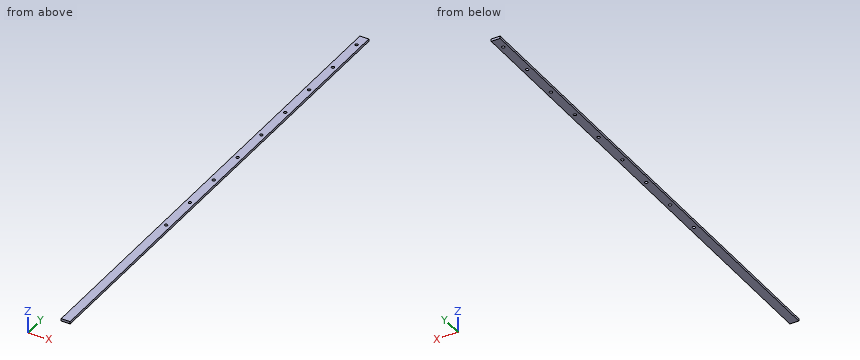
from build123d import *

# Parameters (mm, degrees)
SKETCH1_W           = 18
SKETCH1_H           = 1003
BOSS_EXTRUDE1_DEPTH = 5
SKETCH2_R           = 3
CUT_EXTRUDE1_DEPTH  = 5
LPATTERN1_COUNT     = 9
LPATTERN1_PITCH     = 80


with BuildPart() as part:
    # Sketch1 → Boss-Extrude1 (new body)
    with BuildSketch(Plane.XY):
        Rectangle(SKETCH1_W, SKETCH1_H)
    extrude(amount=BOSS_EXTRUDE1_DEPTH)

    # Sketch2 → Cut-Extrude1 (cut)
    with BuildSketch(Plane.XY.offset(5)):
        with Locations((0, 475.82)):
            Circle(SKETCH2_R)
    cut_extrude1 = extrude(amount=-CUT_EXTRUDE1_DEPTH, mode=Mode.SUBTRACT)

    # LPattern1: Cut-Extrude1 ×9
    with Locations(*[(0, -i * LPATTERN1_PITCH, 0) for i in range(1, LPATTERN1_COUNT)]):
        add(cut_extrude1, mode=Mode.SUBTRACT)


solid = part.part
Read the model definition and answer for the solid it produces. Units are mm, in the model's axes. Round coordinates to 2 decimals unless told otherwise and drop trailing zeros. One line per question, with ' | ' between items. Start each with the question number.
Q1. Find the intervals of material crossed by L1, parallel to X at y = 315.82, z = 3.6; L2, parallel to X at y = 318.5, z = 2.1, in increasing order.
Q2. Section A-A on x = 0 is taken. Count the separate pieces of the cut face and the enclosed holes in it, plus the area to 4 significant figures.
Q3. Flat-ended cylindrical pins translate along their axes: pin 1 (5.5 mm diameter, centred on x = 0, y = -164.18, fed in from +Z); pin 2 (9.5 mm diameter, centred on x = 0, y = 155.82, fed in from +Z). Find the tip coordinate at first contact, or state that the pin passes through.
Established:
1) L1: -9 to -3, 3 to 9 | L2: -9 to -1.35, 1.35 to 9
2) separate pieces: 10 | enclosed holes: 0 | area: 4,745 mm²
3) pin 1: through | pin 2: z = 5
